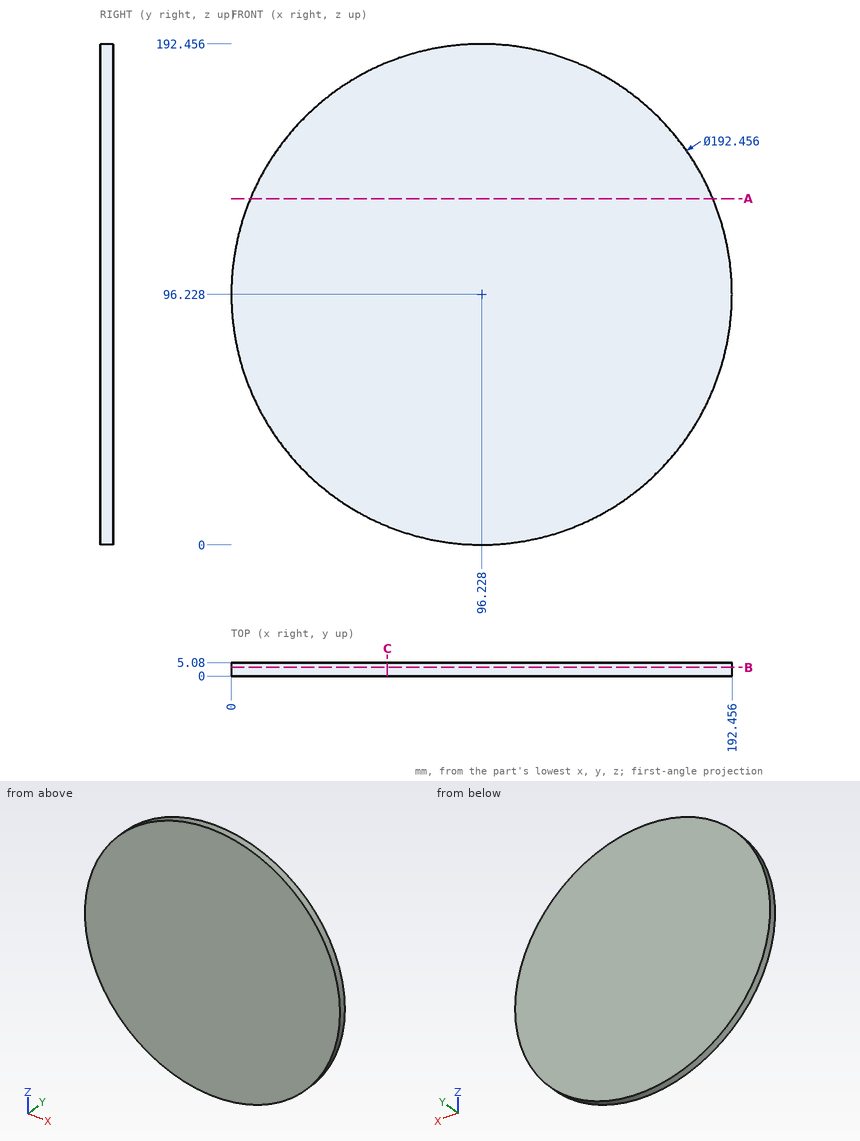
Geometry: see drawing. Coordinates: mm, zero at the bounding-box minimum. Give positions to 0.01 mm unless a question says otherwise; leave off trailing zeros. Order: outer loops, then holes, each group sorted by start corner. A loop starts at its lowest first (then second) coordinate and runs counter-clockwise, first axis right, second up. Notation, with made-up numbers: (52, -24) - (75, -24) arc R6 ccw to (75, -20) - close; hole circle Ø6 at (-18.5, -18). An arc over 180 degrees is marked (long way). Use a Markdown table: item, result.
(1) Line query: line 1 (Z direction, x = 98, y = 3.1); line 2 (Z direction, x = 27, y = 4.9) (1 decimal); line 3 (X direction, y = 2.3, z = 98.5). Output: solid intervals per line, ascending. Write a range as from..to.
Computed values:
| item | result |
|---|---|
| line 1 | z = 0.02..192.44 |
| line 2 | z = 29.4..163.1 |
| line 3 | x = 0.03..192.43 |
(2) Section query A-A (z = 133). Output: boundary loops of the cut face in (x, y).
Computed values:
| item | result |
|---|---|
| outline | (7.3, 0) - (185.15, 0) - (185.15, 5.08) - (7.3, 5.08) - close |
(3) Pin query (flat end, axial travel): pin 1 (1.5 mm diameter, centred on y = 3.5, z = 34, fed in from -X); pin 2 (1.5 mm diameter, centred on y = 4, z = 147, fed in from +X). Return the tip coordinate at first contact, or that it passes through.
Computed values:
| item | result |
|---|---|
| pin 1 | stops at x = 22.2 |
| pin 2 | stops at x = 178.43 |
(4) Section query C-C (x = 60). Output: boundary loops of the cut face in (y, z).
Computed values:
| item | result |
|---|---|
| outline | (0, 7.08) - (5.08, 7.08) - (5.08, 185.38) - (0, 185.38) - close |
(5) Section query B-B (y = 3.35). Output: boundary loops of the cut face in (x, z).
Computed values:
| item | result |
|---|---|
| outline | circle Ø192.46 at (96.23, 96.23) |
